Autodesk Inventor part; units mm, degrees
ref_plane "FRONT" through (0, 0, 0) normal (0, 0, 1) x (1, 0, 0)
ref_plane "TOP" through (0, 0, 0) normal (0, 1, 0) x (-1, 0, 0)
ref_plane "RIGHT" through (0, 0, 0) normal (1, 0, 0) x (0, 1, 0)
ref_plane "FRONT" through (0, 0, 0) normal (0, 0, 1) x (1, 0, 0)
ref_plane "TOP" through (0, 0, 0) normal (0, 1, 0) x (-1, 0, 0)
ref_plane "RIGHT" through (0, 0, 0) normal (1, 0, 0) x (0, 1, 0)
ref_plane "Work Plane4" through (0, 0, 0) normal (0, 0, 1) x (1, 0, 0)
sketch "Sketch1" plane through (0, 0, 0) normal (0, 0, 1) x (1, 0, 0)
  line L0 (3.2, 16) -> (0, 16)
  line L1 (3.2, 3.2) -> (3.2, 14)
  line L2 (3.2, 14) -> (3.2, 16)
  line L3 (0, 16) -> (0, 14)
  line L4 (0, 14) -> (0, 0)
  line L5 (0, 0) -> (14, 0)
  line L6 (16, 0) -> (16, 3.2)
  line L7 (16, 3.2) -> (14, 3.2)
  line L8 (14, 3.2) -> (3.2, 3.2)
  line L9 (14, 0) -> (16, 0)
extrude "Extrusion1" add sketch "Sketch1" along normal blind 80
sketch "Sketch2" plane through (0, 0, 0) normal (-1, 0, 0) x (0, 0, 1)
  circle A0 centre (8, 9.6) radius 1.85
  circle A1 centre (24, 9.6) radius 1.85
  circle A2 centre (40, 9.6) radius 1.85
  circle A3 centre (56, 9.6) radius 1.85
  circle A4 centre (72, 9.6) radius 1.85
  point P0 (0, 0)
hole "Hole1" at (0, 9.6, 8) at (0, 9.6, 24) at (0, 9.6, 40) at (0, 9.6, 56) at (0, 9.6, 72) direction (1, 0, 0) diameter 3.7 end through all
sketch "Sketch3" plane through (0, 0, 0) normal (0, -1, 0) x (1, 0, 0)
  circle A0 centre (9.6, 56) radius 1.85
  circle A1 centre (9.6, 40) radius 1.85
  circle A2 centre (9.6, 24) radius 1.85
  circle A3 centre (9.6, 8) radius 1.85
  circle A4 centre (9.6, 72) radius 1.85
  point P0 (0, 0)
hole "Hole2" at (9.6, 0, 8) at (9.6, 0, 24) at (9.6, 0, 40) at (9.6, 0, 56) at (9.6, 0, 72) direction (0, 1, 0) diameter 3.7 end through all
fillet "Fillet1" radius 2 1 edges at (16, 1.6, 80)
fillet "Fillet2" radius 2 3 edges at (1.6, 16, 80) (1.6, 16, 0) (16, 1.6, 0)
properties part number "inside Angle beam"
The listing builds one solid part. Answer for the finished solid, in the listing's coordinates (mm). A direction names the side the tool comes from. Give positions to 0.01 mm unless a question says otherwise; leave off trailing zeros. Write each loop counter-clockwise with the first axis right and the second up, starting at its lowest first coordinate (ties: lowest second). Pieces come first, ordered by that corner, then holes. Notation, with made-up numbers: (64.25, 0.25) -> (81.25, 0.25) arc R25 cw to (81.25, 37.25) -> close; hole circle Ø6 at (75, 11.25). An arc over 180 degrees is marked (long way). Write item = value, one per line. Start each with the question number.
1) The part is cut by section A-A, the plane x = 9.6. Determine the outline of the cut face in (y, z).
2) The part is cut by section D-D, the plane x = 1. Determine the outline of the cut face in (y, z), and give its area (3 significant figures).
3) Each of these flat-tipped pins is pushed along its axis until it touches: pin 1 (5 mm diameter, centred on x = 12, z = 40, fed in from +Y); pin 2 (2 mm diameter, centred on y = 6.5, z = 71, fed in from +X). Where does it stop, or does it pass through?
4) Which of the six approach directions +Z, -Z, +X, -X, +Y, -Y give full straight-line access (tool end or side, diameter ignored) to faces 5 (the face through (3.2, 7, 39)), 6 (the face through (9.52, 1.62, 57.85))?
5) Determine the mould class of faces 1 (the face through (1.622, 10.726, 70.532)), 2 (the face through (13, 3.2, 39)), 3 (the face through (4, 2, 0)), 4 (the face through (1.62, 9.52, 22.15)) for opening direction Y: +Y half, -Y half, draft (parallel to the pull), parting line (faces both ways), or undercut.
6) The part is cut by section C-C, the plane z = 40. Determine the outline of the cut face in (x, y), and give its area (3 significant figures).
7) Straight lines are drawn through the part: line 1 along Z through (x, y) = (9.6, 1.6); line 2 along Y through (x, z) = (1.7, 40). For each, find the intervals that lie inside material, in ascending order.
Solutions:
q1.outline = (0, 0) -> (3.2, 0) -> (3.2, 6.15) -> (0, 6.15) -> close; (0, 9.85) -> (3.2, 9.85) -> (3.2, 22.15) -> (0, 22.15) -> close; (0, 25.85) -> (3.2, 25.85) -> (3.2, 38.15) -> (0, 38.15) -> close; (0, 41.85) -> (3.2, 41.85) -> (3.2, 54.15) -> (0, 54.15) -> close; (0, 57.85) -> (3.2, 57.85) -> (3.2, 70.15) -> (0, 70.15) -> close; (0, 73.85) -> (3.2, 73.85) -> (3.2, 80) -> (0, 80) -> close
q2.outline = (0, 0) -> (14, 0) arc R2 ccw to (16, 2) -> (16, 78) arc R2 ccw to (14, 80) -> (0, 80) -> close; hole circle Ø3.7 at (9.6, 8); hole circle Ø3.7 at (9.6, 24); hole circle Ø3.7 at (9.6, 40); hole circle Ø3.7 at (9.6, 56); hole circle Ø3.7 at (9.6, 72)
q2.area = 1,220 mm²
q3.pin_1 = 3.2
q3.pin_2 = 3.2
q4.face_5 = +Z, -Z, +X, +Y
q4.face_6 = +Y, -Y
q5.face_1 = undercut
q5.face_2 = +Y half
q5.face_3 = draft
q5.face_4 = undercut
q6.outline = (0, 0) -> (7.75, 0) -> (7.75, 3.2) -> (3.2, 3.2) -> (3.2, 7.75) -> (0, 7.75) -> close; (0, 11.45) -> (3.2, 11.45) -> (3.2, 16) -> (0, 16) -> close; (11.45, 0) -> (16, 0) -> (16, 3.2) -> (11.45, 3.2) -> close
q6.area = 68.5 mm²
q7.line_1 = 0 to 6.15, 9.85 to 22.15, 25.85 to 38.15, 41.85 to 54.15, 57.85 to 70.15, 73.85 to 80
q7.line_2 = 0 to 7.75, 11.45 to 16
